Source: three-view drawing plus pictorial views. Frame: mm from the lowest corner of the part. Give positions to 0.01 mm unless a question says otherwise; leave off trailing zeros. Answer as a JSON object with one key per item and string values. Group by question number.
1) First-contact query: P1, Ø3, axis at x = 5, y = 5, coming from the +Z side. Flat tip, straight axial feed; report the tip coordinate or a pass-through.
2) Ray query, L1, parallel to Y at x = 30, z = 9.5; L2, parallel to Y at x = 5, z = 6.75. Return the intervals inside material, ascending.
3) Section query A-A on z = 4.5. Count the separate pieces of the cut face and the enclosed holes in it, plus the area to 3 significant figures.
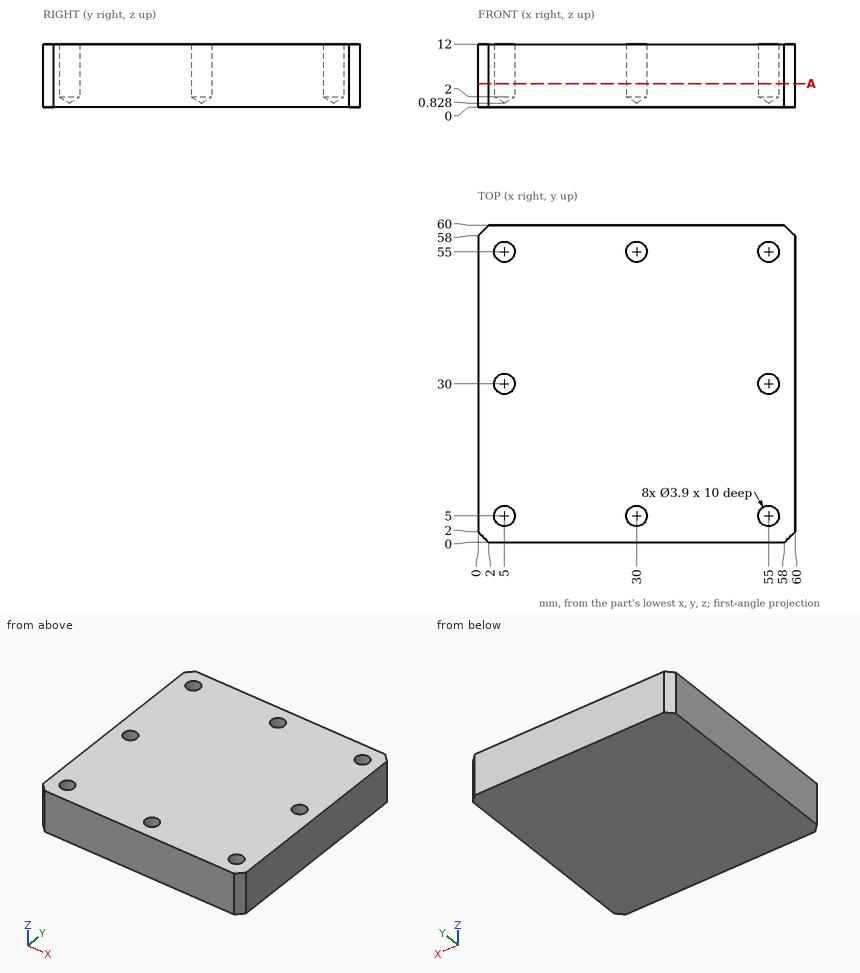
Output:
{
 "1": {"P1": "stops at z = 1.73"},
 "2": {"L1": "y = 0 to 3.05, 6.95 to 53.05, 56.95 to 60", "L2": "y = 0 to 3.05, 6.95 to 28.05, 31.95 to 53.05, 56.95 to 60"},
 "3": {"separate pieces": "1", "enclosed holes": "8", "area": "3,500 mm^2"}
}
